```python
from build123d import *

# Parameters (mm, degrees)
SKETCH1_R           = 3.25
SKETCH1_R_2         = 2.75
SKETCH1_W           = 21
SKETCH1_H           = 40
BOSS_EXTRUDE1_DEPTH = 5
FILLET1_R           = 10
FILLET3_R           = 5
SKETCH3_R           = 2.75
SKETCH3_R_2         = 2.5
CUT_EXTRUDE1_DEPTH  = 10


with BuildPart() as part:
    # Sketch1 → Boss-Extrude1 (new body)
    with BuildSketch(Plane(origin=(0, 0, 0), x_dir=(1, 0, 0), z_dir=(0, 1, 0))):
        with BuildLine():
            ThreePointArc((0, 86.5), (-86.5, 0), (0, -86.5))
            ThreePointArc((0, -86.5), (86.5, 0), (0, 86.5))
        make_face()
        with Locations(Location((-56.214989104, -56.214989104, 0), (0, 0, 270))):
            Circle(SKETCH1_R, mode=Mode.SUBTRACT)
        with Locations(Location((-37, -20.5, 0), (0, 0, 270))):
            Circle(SKETCH1_R_2, mode=Mode.SUBTRACT)
        with Locations(Location((56.214989104, -56.214989104, 0), (0, 0, 270))):
            Circle(SKETCH1_R, mode=Mode.SUBTRACT)
        with Locations(Location((37, -20.5, 0), (0, 0, 270))):
            Circle(SKETCH1_R_2, mode=Mode.SUBTRACT)
        with Locations((-61.5, 0)):
            Rectangle(SKETCH1_W, SKETCH1_H, mode=Mode.SUBTRACT)
        with Locations(Location((-37, 20.5, 0), (0, 0, 270))):
            Circle(SKETCH1_R_2, mode=Mode.SUBTRACT)
        with Locations(Location((-56.214989104, 56.214989104, 0), (0, 0, 270))):
            Circle(SKETCH1_R, mode=Mode.SUBTRACT)
        with BuildLine():
            ThreePointArc((-25, 68.585712798), (0, 73), (25, 68.585712798))
            Line((25, 68.585712798), (25, 20))
            Line((25, 20), (25, -20))
            Line((25, -20), (25, -68.585712798))
            ThreePointArc((25, -68.585712798), (0, -73), (-25, -68.585712798))
            Line((-25, -68.585712798), (-25, -20))
            Line((-25, -20), (-25, 20))
            Line((-25, 20), (-25, 68.585712798))
        make_face(mode=Mode.SUBTRACT)
        with Locations(Location((37, 20.5, 0), (0, 0, 270))):
            Circle(SKETCH1_R_2, mode=Mode.SUBTRACT)
        with Locations((61.5, 0)):
            Rectangle(SKETCH1_W, SKETCH1_H, mode=Mode.SUBTRACT)
        with Locations(Location((56.214989104, 56.214989104, 0), (0, 0, 270))):
            Circle(SKETCH1_R, mode=Mode.SUBTRACT)
    extrude(amount=BOSS_EXTRUDE1_DEPTH)

    # Fillet1
    fillet1_edges = [part.edges().sort_by_distance(p)[0] for p in [
        (72, 2.5, 20),
        (72, 2.5, -20),
        (-72, 2.5, -20),
        (-72, 2.5, 20),
    ]]
    fillet(fillet1_edges, radius=FILLET1_R)

    # Fillet3
    fillet3_edges = [part.edges().sort_by_distance(p)[0] for p in [
        (51, 2.5, -20),
        (51, 2.5, 20),
        (-51, 2.5, -20),
        (-51, 2.5, 20),
    ]]
    fillet(fillet3_edges, radius=FILLET3_R)

    # Sketch3 → Cut-Extrude1 (cut)
    with BuildSketch(Plane(origin=(0, 5, 0), x_dir=(1, 0, 0), z_dir=(0, 1, 0))):
        with Locations(Location((-50.695888728, -36.553753105, 0), (0, 0, 270))):
            Circle(SKETCH3_R)
        with Locations(Location((-36.553753105, -50.695888728, 0), (0, 0, 270))):
            Circle(SKETCH3_R_2)
        with Locations(Location((-36.553753105, 50.695888728, 0), (0, 0, 270))):
            Circle(SKETCH3_R)
        with Locations(Location((-50.695888728, 36.553753105, 0), (0, 0, 270))):
            Circle(SKETCH3_R_2)
        with Locations(Location((50.695888728, 36.553753105, 0), (0, 0, 270))):
            Circle(SKETCH3_R)
        with Locations(Location((36.553753105, 50.695888728, 0), (0, 0, 270))):
            Circle(SKETCH3_R_2)
        with Locations(Location((36.553753105, -50.695888728, 0), (0, 0, 270))):
            Circle(SKETCH3_R)
        with Locations(Location((50.695888728, -36.553753105, 0), (0, 0, 270))):
            Circle(SKETCH3_R_2)
    extrude(amount=-CUT_EXTRUDE1_DEPTH, mode=Mode.SUBTRACT)


solid = part.part
```
Could you check a few things on this model? Use its own coordinates, in mm. Round coordinates to 2 decimals unless told otherwise and drop trailing zeros. Write each loop counter-clockwise with the first axis right and the second up, starting at its lowest first coordinate (ties: lowest second). Pieces come first, ordered by that corner, then holes. Notation, with made-up numbers: M -28.75,30.25 L 19.25,30.25 A27 ccw 19.25,49.25 Z; hole C 75,85 d2. An arc over 180 degrees is marked long. Answer in a Markdown table with one row per item. Add a question column.
Q1. Imagine slicing it at D-D (y = 2.4). Give the number of separate pieces and of enclosed holes in the cut face, then the cut area to 3 significant figures.
Q2. If I drill on line 1 (Z direction, x = -36, y = 2.4); line 2 (X direction, y = 1.9, z = 20.5); line 3 (X direction, y = 2.3, z = 35), over which ranges is the centre line in solid material (lowest first)? Write a range as from..to.
Q3. If we mould it in two halves opening along Z, with no side actions, what happens to faces 1 (the cylindrical face through (-33.13, 2.465, 79.904)), 2 (the cylindrical face through (68.99, 2.54, 17.15))? For each: +Z half, -Z half, draft (parallel to the pull), parting line (faces both ways), or undercut.
Q4. Imagine slicing it at A-A (z = -26). Please give me the cut outline in (x, y).
Q5. Will these pins go through, and if not, where does the flat tip stop? pin 1 Ø2.5 at (x, y) = (-58, 2.5) entering from +Z; pin 2 Ø3 at (y, z) = (2.5, -54.5) entering from +X; pin 3 Ø3 at (x, z) = (-50.7, -36.55) entering from -Y; pin 4 Ø2 at (x, y) = (9, 1.5) entering from -Z.
Q6. Imagine slicing it at B-B (x = -8). Please give me the cut outline in (y, z), then the cut area to 3 significant figures.
Q7. Imagine slicing it at C-C (z = 0). Please give me the cut outline in (x, y), then the cut area to 3 significant figures.
Values:
| question | item | result |
|---|---|---|
| 1 | separate pieces | 1 |
| 1 | enclosed holes | 19 |
| 1 | area | 14,400 mm^2 |
| 2 | line 1 | -78.65..-53.39, -48..-23.06, -17.94..17.94, 23.06..48.26, 53.13..78.65 |
| 2 | line 2 | -84.04..-39.75, -34.25..-25, 25..34.25, 39.75..84.04 |
| 2 | line 3 | -79.1..-52.96, -48.43..-25, 25..48.74, 52.65..79.1 |
| 3 | face 1 | parting line |
| 3 | face 2 | undercut |
| 4 | outline | M -82.5,0 L -25,0 L -25,5 L -82.5,5 Z; M 25,0 L 82.5,0 L 82.5,5 L 25,5 Z |
| 5 | pin 1 | z = 65.28 |
| 5 | pin 2 | x = 68.36 |
| 5 | pin 3 | through |
| 5 | pin 4 | z = -86.13 |
| 6 | outline | M 0,-86.13 L 5,-86.13 L 5,-72.56 L 0,-72.56 Z; M 0,72.56 L 5,72.56 L 5,86.13 L 0,86.13 Z |
| 6 | area | 136 mm^2 |
| 7 | outline | M -86.5,0 L -72,0 L -72,5 L -86.5,5 Z; M -51,0 L -25,0 L -25,5 L -51,5 Z; M 25,0 L 51,0 L 51,5 L 25,5 Z; M 72,0 L 86.5,0 L 86.5,5 L 72,5 Z |
| 7 | area | 405 mm^2 |
